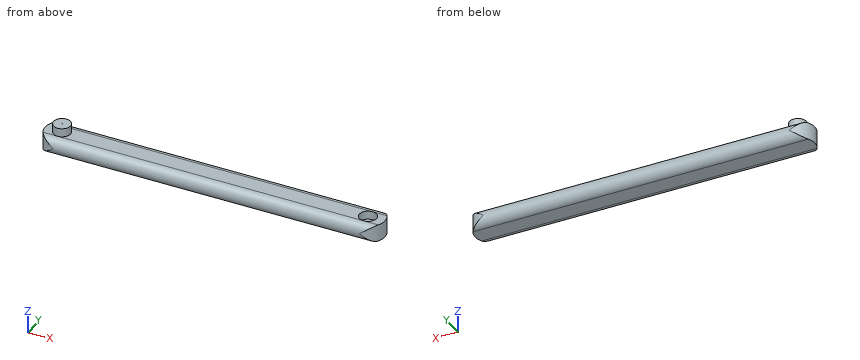
```python
from build123d import *

# Parameters (mm, degrees)
BOSS_EXTRUDE1_DEPTH = 2000
CUT_EXTRUDE1_DEPTH  = 100
SKETCH3_R           = 50
CUT_EXTRUDE2_DEPTH  = 50
SKETCH4_R           = 50
BOSS_EXTRUDE2_DEPTH = 50
SKETCH5_W           = 1.860422616
SKETCH5_H           = 2.197438595
CUT_EXTRUDE3_DEPTH  = 1


with BuildPart() as part:
    # Sketch1 → Boss-Extrude1 (new body)
    with BuildSketch(Plane(origin=(0, 0, 0), x_dir=(0, 0, -1), z_dir=(1, 0, 0))):
        with BuildLine():
            Line((-50, 50), (-50, -50))
            ThreePointArc((-50, -50), (0, -100), (50, -50))
            Line((50, -50), (50, 50))
            ThreePointArc((50, 50), (0, 100), (-50, 50))
        make_face()
    extrude(amount=-BOSS_EXTRUDE1_DEPTH)

    # Sketch2 → Cut-Extrude1 (cut)
    with BuildSketch(Plane.XY.offset(50)):
        with BuildLine():
            Line((-1899.5, 100), (-2000, 100))
            Line((-2000, 100), (-2000, -100))
            Line((-2000, -100), (-1899.5, -100))
            ThreePointArc((-1899.5, -100), (-1999.5, 0), (-1899.5, 100))
        make_face()
        with BuildLine():
            Line((-100.5, 100), (0, 100))
            Line((0, 100), (0, -100))
            Line((0, -100), (-100.5, -100))
            ThreePointArc((-100.5, -100), (-0.5, 0), (-100.5, 100))
        make_face()
    extrude(amount=-CUT_EXTRUDE1_DEPTH, mode=Mode.SUBTRACT)

    # Sketch3 → Cut-Extrude2 (cut)
    with BuildSketch(Plane.XY.offset(50)):
        with Locations((-100, 0)):
            Circle(SKETCH3_R)
    extrude(amount=-CUT_EXTRUDE2_DEPTH, mode=Mode.SUBTRACT)

    # Sketch4 → Boss-Extrude2 (add)
    with BuildSketch(Plane.XY.offset(50)):
        with Locations(Location((-1899.5, 0, 0), (0, 0, 270))):
            Circle(SKETCH4_R)
    extrude(amount=BOSS_EXTRUDE2_DEPTH)

    # Sketch5 → Cut-Extrude3 (cut)
    with BuildSketch(Plane.XY.offset(100)):
        with Locations((-1898.569788692, -1.098719297)):
            Rectangle(SKETCH5_W, SKETCH5_H)
    extrude(amount=-CUT_EXTRUDE3_DEPTH, mode=Mode.SUBTRACT)


solid = part.part
```
Could you check a few things on this model? Use its own coordinates, in mm. Round coordinates to 2 decimals unless told otherwise and drop trailing zeros. Write each loop counter-clockwise with the first axis right and the second up, starting at its lowest first coordinate (ties: lowest second). Pieces come first, ordered by that corner, then holes. Notation, with made-up numbers: M 56,-3.75 L 107,-3.75 A14 ccw 107,20.25 Z; hole C 64,88.25 d3. An arc over 180 degrees is marked long. Write each question's results on one line, items separated by ' | '. Start each with the question number.
1. I'm going to push flat-ended pins straight in: pin 1 Ø12 at (y, z) = (20, 80.5) entering from -X; pin 2 Ø1.5 at (x, z) = (-740, -29.5) entering from -Y; pin 3 Ø0.6 at (x, y) = (-1899, -1.5) entering from +Z. Where does each tip first touch, or does it pass through?
2. I need wall thicknesses on L1, parallel to X at y = 0, z = 35; L2, parallel to Z at x = -736, y = -52; L3, parallel to Y at x = -428, z = -3.5. Which ranges of each line are inside material? Lowest first, please. Write a range as from..to.
3. Imagine slicing it at D-D on y = -73. List the corners of the cut face in (x, z) for me, and give its area (3 significant figures).
4. Imagine slicing it at C-C on x = -959. List the corners of the cut face in (y, z) for me.
5. Imagine slicing it at B-B on y = 24.5. List the corners of the cut face in (x, z) for me.
6. Imagine slicing it at A-A on z = 28.5. List the corners of the cut face in (x, y) for me, and give its area (3 significant figures).
Result sheet:
1) pin 1: stops at x = -1947.5 | pin 2: stops at y = -90.91 | pin 3: stops at z = 99
2) L1: x = -1999.5..-150, -50..-0.5 | L2: z = -49.96..49.96 | L3: y = -99.88..99.88
3) outline: M -1967.84,-44.4 L -32.16,-44.4 L -32.16,44.4 L -1967.84,44.4 Z | area: 172,000 mm^2
4) outline: M -50,-50 L 50,-50 A50 ccw 50,50 L -50,50 A50 ccw Z
5) outline: M -1996.45,-50 L -3.55,-50 L -3.55,50 L -56.41,50 L -56.41,0 L -143.59,0 L -143.59,50 L -1855.91,50 L -1855.91,100 L -1943.09,100 L -1943.09,50 L -1996.45,50 Z
6) outline: M -1940.78,-91.08 L -59.22,-91.08 A100 ccw -59.22,91.08 L -1940.78,91.08 A100 ccw Z; hole C -100,0 d100 | area: 350,000 mm^2
